Geometry check sheet. Reference: the model listing, model coordinates, mm. Give positions to 0.01 mm unless a question says otherwise; leave off trailing zeros. Write each loop counter-clockwise with the first axis right and the second up, starting at its lowest first coordinate (ties: lowest second). Pieces come first, ordered by that corner, then holes. Notation, with made-up numbers: (-27.75, 75) - (28.25, 75) arc R7 ccw to (28.25, 87) - close; hole circle Ø3 at (57.25, 65.25). An arc over 180 degrees is marked (long way). Use a Markdown table: item, result.
Autodesk Inventor part; units mm, degrees
ref_plane "YZ Plane" through (0, 0, 0) normal (1, 0, 0) x (0, 1, 0)
ref_plane "XZ Plane" through (0, 0, 0) normal (0, 1, 0) x (-1, 0, 0)
ref_plane "XY Plane" through (0, 0, 0) normal (0, 0, 1) x (1, 0, 0)
sketch "Sketch1" plane through (0, 0, 0) normal (0, 1, 0) x (-1, 0, 0)
  arc A0 (3.5, 0) -> (-3.5, 0) centre (0, 0) ccw
  arc A1 (-3.5, -85) -> (3.5, -85) centre (0, -85) ccw
  line L0 (3.5, 0) -> (3.5, -85)
  line L1 (-3.5, 0) -> (-3.5, -85)
  dimension "d0" = 7
  dimension "d1" = 7
  dimension "d9" = 85
extrude "Extrusion1" add sketch "Sketch1" along normal blind 3
sketch "Sketch2" plane through (0, 3, 0) normal (0, 1, 0) x (1, 0, 0)
  circle A0 centre (0, 0) radius 2
  circle A1 centre (0, 85) radius 2
  arc A2 (3.5, 85) -> (-3.5, 85) centre (0, 85) ccw
  dimension "d4" = 4
  dimension "d5" = 4
  dimension "d10" = 1.5
extrude "Extrusion2" cut sketch "Sketch2" against normal blind 3
properties part number "tay quay"
1) Mould release check, pull along X, two halves, no side actions. Record for faces 1 (the cylindrical face through (0, 2, -87)), 2 (the cylindrical face through (0.1, 1.5, 3.5)), 3 (the flat face through (3.5, 1, -42)): pulls with the +X half, pulls with the -X half, needs draft (parallel to the pull), parting line crosses it, or undercut.
Working result:
| item | result |
|---|---|
| face 1 | undercut |
| face 2 | parting line crosses it |
| face 3 | pulls with the +X half |
2) Section check B-B on y = 1. Record the boundary of the cut face in (x, z).
Working result:
| item | result |
|---|---|
| outline | (-3.5, -85) arc R3.5 ccw to (3.5, -85) - (3.5, 0) arc R3.5 ccw to (-3.5, 0) - close; hole circle Ø4 at (0, -85); hole circle Ø4 at (0, 0) |
3) Section check A-A on x = 0. Record the boundary of the cut face in (y, z).
Working result:
| item | result |
|---|---|
| outline | (0, -88.5) - (3, -88.5) - (3, -87) - (0, -87) - close; (0, -83) - (3, -83) - (3, -2) - (0, -2) - close; (0, 2) - (3, 2) - (3, 3.5) - (0, 3.5) - close |
4) Depth check by flat-ended pin: P1, Ø1.5, axis at x = 1.5, y = 2, coming from the -Z side. Enter the tip coordinate at first touch or a pass-through.
Working result:
| item | result |
|---|---|
| P1 | stops at z = -88.42 |
5) Material ranges on L1, parallel to Z at x = 0, y = 1.35; L2, parallel to X at y = 1.8, z = -85; L3, parallel to Z at x = -1, y = 1.8, recorded low to high. Write a range as from..to.
Working result:
| item | result |
|---|---|
| L1 | z = -88.5..-87, -83..-2, 2..3.5 |
| L2 | x = -3.5..-2, 2..3.5 |
| L3 | z = -88.35..-86.73, -83.27..-1.73, 1.73..3.35 |
